from build123d import *

# Parameters (mm, degrees)
SKETCH_1_R               = 15
SKETCH_1_R_2             = 2.5
EXTRUDE_1_DEPTH          = 3
SKETCH_2_R               = 1
EXTRUDE_2_DEPTH          = 10
PATTERN_CIRCULAR_1_COUNT = 15
EXTRUDE_START            = 10
SKETCH_3_R               = 1
EXTRUDE_3_DEPTH          = 10
PATTERN_CIRCULAR_2_COUNT = 5


with BuildPart() as part:
    # 草圖1 → 填料-伸長1 (new body)
    with BuildSketch(Plane(origin=(0, 0, 0), x_dir=(1, 0, 0), z_dir=(0, 1, 0))):
        with Locations(Location((0, 0, 0), (0, 0, 270))):
            Circle(SKETCH_1_R)
        with Locations(Location((0, 0, 0), (0, 0, 270))):
            Circle(SKETCH_1_R_2, mode=Mode.SUBTRACT)
    extrude(amount=EXTRUDE_1_DEPTH)

    # 草圖2 → 填料-伸長2 (add)
    with BuildSketch(Plane(origin=(0, 3, 0), x_dir=(1, 0, 0), z_dir=(0, 1, 0))):
        with Locations(Location((12.4808724, -0.691248248, 0), (0, 0, 270))):
            Circle(SKETCH_2_R)
    extrude_2 = extrude(amount=EXTRUDE_2_DEPTH)

    # 環狀複製排列1: 填料-伸長2 ×15 about axis
    pattern_circular_1_axis = Axis((0, 0, 0), (0, 1, 0))
    for i in range(1, PATTERN_CIRCULAR_1_COUNT):
        add(extrude_2.rotate(pattern_circular_1_axis, i * 360 / PATTERN_CIRCULAR_1_COUNT))

    # 草圖3 → 填料-伸長3 (add)
    with BuildSketch(Plane.XZ.offset(EXTRUDE_START)):
        with Locations(Location((12.4808724, 0.691248248, 0), (0, 0, 90))):
            Circle(SKETCH_3_R)
    extrude_3 = extrude(amount=-EXTRUDE_3_DEPTH)

    # 環狀複製排列2: 填料-伸長3 ×5 about axis
    pattern_circular_2_axis = Axis((0, 0, 0), (0, 1, 0))
    for i in range(1, PATTERN_CIRCULAR_2_COUNT):
        add(extrude_3.rotate(pattern_circular_2_axis, i * 360 / PATTERN_CIRCULAR_2_COUNT))


solid = part.part
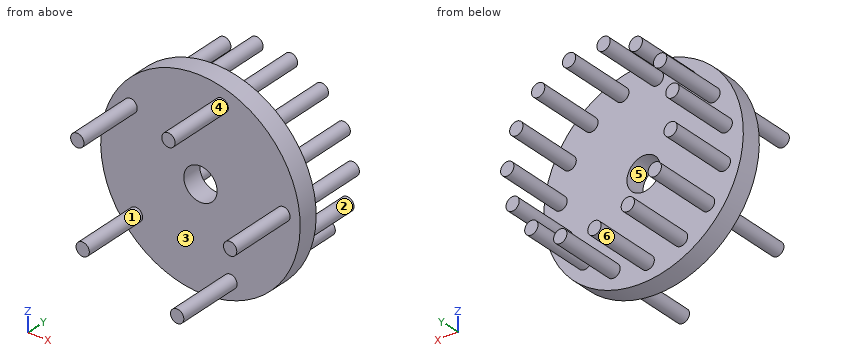
The listing builds one solid part. Answer for the finished solid, in the listing's coordinates (mm). Face numbers are marked on the shaded views. A direction names the side the tool comes from. Coordinates: 2 decimals unless noted, no trailing zeros. Order: outer loops, then holes, each group sorted by start corner. A loop starts at its lowest first (then second) coordinate and runs counter-clockwise, first axis right, second up.
Q1. Consider line 1 (X direction, y = 1.25, z = 0); line 2 (Y direction, x = -11.75, z = -5.75); line 3 (Z direction, x = 12.5, y = -5.5). Determine where each line is inside the solid, lowest interval first.
Q2. Given P1, Ø1, axis at x = -1, y = 0, coming from the -Z side; P2, Ø8, axis at x = -10, y = -6, coming from the +Z side; P3, Ø9, axis at x = -7, z = -3, coming from the -Y side; P4, Ø12, axis at x = 4, y = 6.5, coming from the +Z side, each flat-ended and moving along its own axis, determine where each tip first touches the part or whether it passes through.
Q3. A cutting plane is placed at C-C, the plane y = 2. Write down the section's boundary in (x, z).
Q4. A cutting plane is placed at B-B, the plane y = -8. Write down the section's boundary in (x, z).
Q5. A cutting plane is placed at A-A, the plane z = -1.5. Write down the section's boundary in (x, y).
Q6. For a pull along X with two mould halves and no side action, classify the marked faces 1, 2 and 3 as pulls with the +X half, pulls with the -X half, needs draft (parallel to the pull), parting line crosses it, or undercut.
Q7. Which of the six approach directions +Z, -Z, +X, -X, +Y, -Y give full straight-line access (tool end or side, diameter ignored) to the marked faces 4, 5 and 6?
Answers follow:
1. line 1: x = -15 to -2.5, 2.5 to 15
1. line 2: y = 0 to 3
1. line 3: z = -0.31 to 1.69
2. P1: stops at z = -14.99
2. P2: stops at z = 7.78
2. P3: stops at y = 0
2. P4: stops at z = 15
3. outline: circle Ø30 at (0, 0); hole circle Ø5 at (0, 0)
4. outline: circle Ø2 at (-10.5, 6.78); circle Ø2 at (-9.69, -7.9); circle Ø2 at (3.2, 12.08); circle Ø2 at (4.51, -11.66); circle Ø2 at (12.48, 0.69)
5. outline: (-14.92, 0) - (-2, 0) - (-2, 3) - (-14.92, 3) - close; (2, 0) - (14.92, 0) - (14.92, 3) - (2, 3) - close
6. face 1: parting line crosses it
6. face 2: undercut
6. face 3: needs draft
7. face 4: -Y
7. face 5: +Y, -Y
7. face 6: +Y
